Read the model definition and answer for the solid it produces. Units are mm, in the model's axes. Give positions to 0.01 mm unless a question says otherwise; leave off trailing zeros. Order: outer loops, then holes, each group sorted by start corner. A loop starts at its lowest first (then second) coordinate and runs counter-clockwise, first axis right, second up. Notation, with made-up numbers: (-25, -33.5) -> (34, -33.5) arc R20 cw to (34, -26.5) -> close; hole circle Ø3 at (-15.5, 66.5). An arc over 180 degrees is marked (long way). Answer as CSV lines item,"result". Start each with the question number.
1) Find section C-C (x = -233). Determine the outline of the cut face in (y, z) (3 decimals), and give its area (3 significant figures).
2) Flat-ended cylindrical pins translate along their axes: pin 1 Ø1.6 at (y, z) = (2, 212) entering from -X; pin 2 Ø1.6 at (x, y) = (178.5, 1.5) entering from +Z; pin 3 Ø1 at (x, y) = (327, 2.5) entering from -Z. Find the tip coordinate at first contact, or state that the pin passes through.
3) Find section B-B (x = 196). Determine the outline of the cut face in (y, z) (3 decimals), and give its area (3 significant figures).
4) Find section A-A (y = 1.45). Determine the outline of the cut face in (x, z), and give its area (3 significant figures).
5) Straight lines are drawn through the part: L1, parallel to Z at x = 140.5, y = 2.85; L2, parallel to Z at x = 313.5, y = 2.65; L3, parallel to X at y = 1.85, z = -309. For each, find the intervals that lie inside material, in ascending order. Write a range as from..to.
```python
from build123d import *

# Parameters (mm, degrees)
SKETCH1_W           = 698.5
SKETCH1_H           = 685.8
BOSS_EXTRUDE1_DEPTH = 3.175
CUT_EXTRUDE1_DEPTH  = 4.175
CUT_EXTRUDE2_DEPTH  = 4.175


with BuildPart() as part:
    # Sketch1 → Boss-Extrude1 (new body)
    with BuildSketch(Plane(origin=(0, 0, 0), x_dir=(1, 0, 0), z_dir=(0, 1, 0))):
        Rectangle(SKETCH1_W, SKETCH1_H)
    extrude(amount=BOSS_EXTRUDE1_DEPTH)

    # Sketch3 → Cut-Extrude1 (cut, through all)
    with BuildSketch(Plane(origin=(0, 3.175, 0), x_dir=(1, 0, 0), z_dir=(0, 1, 0))):
        Polygon((-298.45, 203.2), (-209.55, 292.1), (-209.55, 342.9), (-349.25, 342.9), (-349.25, 203.2), align=None)
        Polygon((-349.25, -203.2), (-298.45, -203.2), (-209.55, -292.1), (-209.55, -342.9), (-349.25, -342.9), align=None)
        Polygon((349.25, 203.2), (298.45, 203.2), (209.55, 292.1), (209.55, 342.9), (349.25, 342.9), align=None)
    extrude(amount=-CUT_EXTRUDE1_DEPTH, mode=Mode.SUBTRACT)

    # Sketch7 → Cut-Extrude2 (cut, through all)
    with BuildSketch(Plane(origin=(-6.096, 3.175, 0.254), x_dir=(1, 0, 0), z_dir=(0, 1, 0))):
        Polygon((133.096, -190.5), (133.096, -355.346), (368.046, -355.346), (368.046, -209.55), (329.946, -209.55), (329.946, -241.046), (228.346, -241.046), (228.346, -190.5), align=None)
    extrude(amount=-CUT_EXTRUDE2_DEPTH, mode=Mode.SUBTRACT)


solid = part.part
```
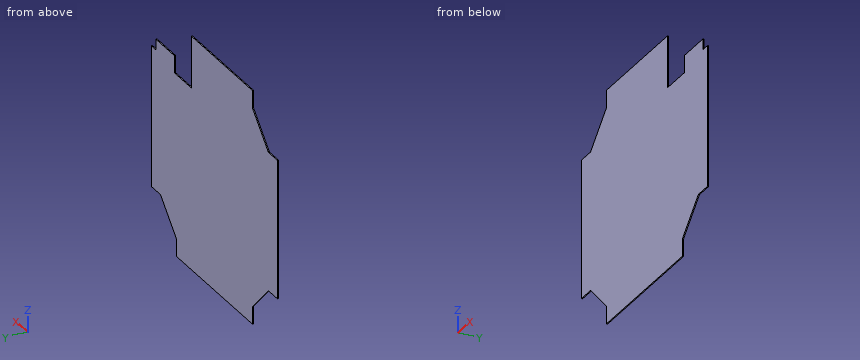
Findings below:
1,outline,"(0, -268.65) -> (3.175, -268.65) -> (3.175, 268.65) -> (0, 268.65) -> close"
1,area,"1,710 mm²"
2,pin 1,"x = -290.45"
2,pin 2,"z = 190.75"
2,pin 3,"z = -203.2"
3,outline,"(0, -342.9) -> (3.175, -342.9) -> (3.175, 190.754) -> (0, 190.754) -> close"
3,area,"1,690 mm²"
4,outline,"(-349.25, -203.2) -> (-298.45, -203.2) -> (-209.55, -292.1) -> (-209.55, -342.9) -> (209.55, -342.9) -> (209.55, -292.1) -> (298.45, -203.2) -> (349.25, -203.2) -> (349.25, 209.8) -> (323.85, 209.8) -> (323.85, 241.3) -> (222.25, 241.3) -> (222.25, 190.75) -> (127, 190.75) -> (127, 342.9) -> (-209.55, 342.9) -> (-209.55, 292.1) -> (-298.45, 203.2) -> (-349.25, 203.2) -> close"
4,area,"404,000 mm²"
5,L1,"-342.9..190.75"
5,L2,"-203.2..241.3"
5,L3,"-209.55..209.55"
